```python
from build123d import *

# Parameters (mm, degrees)
SKETCH1_R               = 1.5
SKETCH1_R_2             = 5
SKETCH1_R_3             = 2.5
BOSS_EXTRUDE1_DEPTH     = 3.2
FILLET1_R               = 30
CHAMFER1_SIZE           = 5
CUT_EXTRUDE1_REACH      = 347.919
CUT_EXTRUDE1_END_RADIUS = 25
SKETCH3_R               = 2.5


with BuildPart() as part:
    # Sketch1 → Boss-Extrude1 (new, symmetric)
    with BuildSketch(Plane.XY):
        with BuildLine():
            Line((345, 19.05), (16.189425561, 19.05))
            ThreePointArc((16.189425561, 19.05), (-25, 0), (16.189425561, -19.05))
            Line((16.189425561, -19.05), (345, -19.05))
            Line((345, -19.05), (345, 19.05))
        make_face()
        with Locations((8.980256121, 8.980256121)):
            Circle(SKETCH1_R, mode=Mode.SUBTRACT)
        Circle(SKETCH1_R_2, mode=Mode.SUBTRACT)
        with Locations((330, 0)):
            Circle(SKETCH1_R_3, mode=Mode.SUBTRACT)
        with Locations((310, 0)):
            Circle(SKETCH1_R_3, mode=Mode.SUBTRACT)
        with Locations((290, 0)):
            Circle(SKETCH1_R_3, mode=Mode.SUBTRACT)
        with Locations((270, 0)):
            Circle(SKETCH1_R_3, mode=Mode.SUBTRACT)
        with Locations((250, 0)):
            Circle(SKETCH1_R_3, mode=Mode.SUBTRACT)
        with Locations((230, 0)):
            Circle(SKETCH1_R_3, mode=Mode.SUBTRACT)
        with Locations((210, 0)):
            Circle(SKETCH1_R_3, mode=Mode.SUBTRACT)
        with Locations((190, 0)):
            Circle(SKETCH1_R_3, mode=Mode.SUBTRACT)
        with Locations((8.980256121, -8.980256121)):
            Circle(SKETCH1_R, mode=Mode.SUBTRACT)
        with Locations((-8.980256121, -8.980256121)):
            Circle(SKETCH1_R, mode=Mode.SUBTRACT)
        with Locations((-8.980256121, 8.980256121)):
            Circle(SKETCH1_R, mode=Mode.SUBTRACT)
    extrude(amount=BOSS_EXTRUDE1_DEPTH, both=True)

    # Fillet1
    fillet1_edges = [part.edges().sort_by_distance(p)[0] for p in [
        (16.189425561, -19.05, 0),
        (16.189425561, 19.05, 0),
    ]]
    fillet(fillet1_edges, radius=FILLET1_R)

    # Chamfer1
    chamfer1_edges = [part.edges().sort_by_distance(p)[0] for p in [
        (345, -19.05, 0),
        (345, 19.05, 0),
    ]]
    chamfer(chamfer1_edges, length=CHAMFER1_SIZE)

    # Cut-Extrude1: up to this cylinder (the profile starts inside it)
    cut_extrude1_end = Plane(origin=(0, 0, 0), z_dir=(0, 0, -1)) * Cylinder(CUT_EXTRUDE1_END_RADIUS, 746.838, mode=Mode.PRIVATE)
    # Sketch3 → Cut-Extrude1 (cut, up to the surface)
    with BuildSketch(Plane(origin=(0, 0, 0), x_dir=(0, 0, -1), z_dir=(1, 0, 0)), mode=Mode.PRIVATE) as cut_extrude1_sk1:
        Circle(SKETCH3_R)
    cut_extrude1_tool1 = extrude(cut_extrude1_sk1.sketch, amount=-CUT_EXTRUDE1_REACH, mode=Mode.PRIVATE) & cut_extrude1_end
    add(cut_extrude1_tool1.solids().sort_by_distance((0, 0, 0))[0], mode=Mode.SUBTRACT)


solid = part.part
```
Check sheet for the modelled part. Datum: model origin and axes. Units: mm. A direction names the side the tool comes from. Round coordinates to 2 decimals unless told otherwise and drop trailing zeros. Write each loop counter-clockwise with the first axis right and the second up, starting at its lowest first coordinate (ties: lowest second). Pieces come first, ordered by that corner, then holes. Notation, with made-up numbers: M 50,48 L 105,48 A19 ccw 105,55 Z; hole C 32,-11 d11. An arc over 180 degrees is marked long. Write item = value, one per line. Start each with the question number.
1. Section check C-C, the plane x = 220.5. Record the cut outline in (y, z).
2. Tool access check on faces 1 (the flat face through (345, 0, 0)), 2 (the flat face through (180, -19.05, 0)), 3 (the flat face through (185, 19.05, 0)). Record the directions out of +Z, -Z, +X, -X, +Y, -Y that give a thin tool (end or side, any length) a straight path to the whole face; none if there is none.
3. Gauge pin test, flat ends, axial feed: pin 1 (3 mm diameter, centred on x = 310, y = 0, fed in from -Z); pin 2 (1 mm diameter, centred on y = -12.5, z = 0, fed in from -X); pin 3 (1 mm diameter, centred on y = -3.5, z = -0.5, fed in from -X). Record the tip position at first contact, or that the pin passes through.
4. Scan lines: line 1 (Y direction, x = 0, z = 0.5); line 2 (Z direction, x = -9.5, y = 0); line 3 (Y direction, x = 290, z = 1.75). Record each from-to range of solid material in increasing order. Write a range as [from, to].
5. Release check for a two-part mould opening along X. For faces 4 (the flat face through (157, 0, 3.2)), 5 (the cylindrical face through (4.77, 1.5, -0.04)), 6 (the cylindrical face through (18, 19.85, 0.04)) record: pulls with the +X half, pulls with the -X half, needs draft (parallel to the pull), parting line crosses it, or undercut.
6. Section check B-B, the plane z = -1.25. State how many separate pieces and enclosed holes the cut face has, then the cut area to 3 significant figures.
7. Section check A-A, the plane x = 0. Record the cut outline in (y, z).
Results found:
q1.outline = M -19.05,-3.2 L 19.05,-3.2 L 19.05,3.2 L -19.05,3.2 Z
q2.face_1 = +Z, -Z, +X, +Y, -Y
q2.face_2 = +Z, -Z, +X, -Y
q2.face_3 = +Z, -Z, +X, +Y
q3.pin_1 = through
q3.pin_2 = -21.93
q3.pin_3 = -24.82
q4.line_1 = [-25, -5], [5, 25]
q4.line_2 = [-3.2, -2.5], [2.5, 3.2]
q4.line_3 = [-19.05, -2.5], [2.5, 19.05]
q5.face_4 = needs draft
q5.face_5 = undercut
q5.face_6 = pulls with the +X half
q6.separate_pieces = 1
q6.enclosed_holes = 12
q6.area = 13,900 mm^2
q7.outline = M -25,-3.2 L -5,-3.2 L -5,3.2 L -25,3.2 Z; M 5,-3.2 L 25,-3.2 L 25,3.2 L 5,3.2 Z
